Can you work these out from the model? Positions are in its coordinate system, mm. A direction names the side the tool comes from. Round coordinates to 2 decimals unless told otherwise and drop trailing zeros. Loops run counter-clockwise (first coordinate to the right, second up) from the corner with the lowest first, then second, coordinate; pieces in that order, holes last. Notation, with made-up numbers: (-32.75, -5.75) -> (-6.75, -5.75) arc R21 ccw to (-6.75, 27.25) -> close; hole circle Ø10 at (-15.5, 41.25). An arc over 180 degrees is marked (long way). Write item = value, one per line.
from build123d import *

# Parameters (mm, degrees)
GENERAL_SHAPE_DEPTH      = 800
SKETCH5_W                = 1800
SKETCH5_H                = 700
CUT_EXTRUDE2_DEPTH       = 75
SKETCH6_W                = 1300
SKETCH6_H                = 156.02
WEIGHT_REDUCTION_DEPTH   = 1223.94273789
BOSS_EXTRUDE3_DEPTH      = 900
BOSS_EXTRUDE3_DEPTH_BACK = 900
SKETCH8_W                = 50
SKETCH8_H                = 75
BOSS_EXTRUDE4_DEPTH      = 120
BOSS_EXTRUDE5_DEPTH      = 120
CUT_EXTRUDE4_DEPTH       = 740
CUT_EXTRUDE4_DEPTH_BACK  = 40
SKETCH7_R                = 7.5
BOSS_EXTRUDE6_DEPTH      = 25
BOSS_EXTRUDE6_DEPTH_BACK = 25
SKETCH12_R               = 9.525
SKETCH13_W               = 31.75
SKETCH13_H               = 68.5
CUT_EXTRUDE5_DEPTH       = 1371.819167563


with BuildPart() as part:
    # Sketch1 → General shape (new body)
    with BuildSketch(Plane.XY):
        Polygon((-900, 213.515667244), (900, 213.515667244), (900, -67.504332756), (500, -67.504332756), (-500, -67.504332756), (-900, -67.504332756), align=None)
    extrude(amount=GENERAL_SHAPE_DEPTH)

    # Sketch5 → Cut-Extrude2 (cut)
    with BuildSketch(Plane(origin=(0, 213.515667244, 0), x_dir=(1, 0, 0), z_dir=(0, 1, 0))):
        with Locations((0, -400)):
            Rectangle(SKETCH5_W, SKETCH5_H)
    extrude(amount=-CUT_EXTRUDE2_DEPTH, mode=Mode.SUBTRACT)

    # Sketch6 → Weight reduction (cut, through all)
    with BuildSketch(Plane(origin=(0, 0, 0), x_dir=(-1, 0, 0), z_dir=(0, 0, -1))):
        with Locations((0, 10.505667244)):
            Rectangle(SKETCH6_W, SKETCH6_H)
    extrude(amount=-WEIGHT_REDUCTION_DEPTH, mode=Mode.SUBTRACT)

    # Sketch8 → Boss-Extrude3 (add, two sides: drawn at the far end of the back side and taken through both)
    with BuildSketch(Plane(origin=(0, 0, 0), x_dir=(0, 0, -1), z_dir=(1, 0, 0)).offset(-BOSS_EXTRUDE3_DEPTH_BACK)):
        with Locations((-715, 176.015667244)):
            Rectangle(SKETCH8_W, SKETCH8_H)
        with Locations((-85, 176.015667244)):
            Rectangle(SKETCH8_W, SKETCH8_H)
    extrude(amount=BOSS_EXTRUDE3_DEPTH + BOSS_EXTRUDE3_DEPTH_BACK)

    # Sketch9 → Boss-Extrude4 (add)
    with BuildSketch(Plane(origin=(900, 0, 0), x_dir=(0, 0, -1), z_dir=(1, 0, 0))):
        Polygon((-800, 213.515667244), (-750, 213.515667244), (-750, 138.515667244), (-740, 138.515667244), (-740, 213.515667244), (-690, 213.515667244), (-690, 107.495667244), (-110, 107.495667244), (-110, 182.495667244), (-60, 182.495667244), (-60, 107.495667244), (-50, 107.495667244), (-50, 182.495667244), (0, 182.495667244), (0, -67.504332756), (-800, -67.504332756), align=None)
    extrude(amount=BOSS_EXTRUDE4_DEPTH)

    # Sketch10 → Boss-Extrude5 (add)
    with BuildSketch(Plane.ZY.offset(900)):
        Polygon((800, 213.515667244), (750, 213.515667244), (750, 138.515667244), (740, 138.515667244), (740, 213.515667244), (690, 213.515667244), (690, 107.495667244), (110, 107.495667244), (110, 182.495667244), (60, 182.495667244), (60, 107.495667244), (50, 107.495667244), (50, 182.495667244), (0, 182.495667244), (0, -67.504332756), (800, -67.504332756), align=None)
    extrude(amount=BOSS_EXTRUDE5_DEPTH)

    # Sketch7 → Cut-Extrude4 (cut, two sides: drawn at the far end of the back side and taken through both)
    with BuildSketch(Plane(origin=(0, 0, 750), x_dir=(-1, 0, 0), z_dir=(0, 0, -1)).offset(-CUT_EXTRUDE4_DEPTH_BACK)):
        with Locations(Location((-35, 176.015667244, 0), (0, 0, 180))):
            Circle(SKETCH7_R)
        with Locations(Location((-350, 176.015667244, 0), (0, 0, 180))):
            Circle(SKETCH7_R)
        with Locations(Location((-310, 176.015667244, 0), (0, 0, 180))):
            Circle(SKETCH7_R)
        with Locations(Location((10, 176.015667244, 0), (0, 0, 180))):
            Circle(SKETCH7_R)
        with BuildLine():
            Line((960, 168.515667244), (510, 168.515667244))
            ThreePointArc((510, 168.515667244), (502.5, 176.015667244), (510, 183.515667244))
            Line((510, 183.515667244), (960, 183.515667244))
            ThreePointArc((960, 183.515667244), (967.5, 176.015667244), (960, 168.515667244))
        make_face()
        with BuildLine():
            Line((-1000, 183.515667244), (-675, 183.515667244))
            ThreePointArc((-675, 183.515667244), (-667.5, 176.015667244), (-675, 168.515667244))
            Line((-675, 168.515667244), (-1000, 168.515667244))
            ThreePointArc((-1000, 168.515667244), (-1007.5, 176.015667244), (-1000, 183.515667244))
        make_face()
    extrude(amount=CUT_EXTRUDE4_DEPTH + CUT_EXTRUDE4_DEPTH_BACK, mode=Mode.SUBTRACT)

    # Sketch12 → Boss-Extrude6 (add, two sides: drawn at the far end of the back side and taken through both)
    # profile 1 of 2: a face of its own
    with BuildSketch(Plane(origin=(0, 0, 400), x_dir=(-1, 0, 0), z_dir=(0, 0, -1)).offset(-BOSS_EXTRUDE6_DEPTH_BACK)):
        with BuildLine():
            Line((72.5, 138.515667244), (72.5, 194.615667244))
            ThreePointArc((72.5, 194.615667244), (68.868124087, 203.383791331), (60.1, 207.015667244))
            Line((60.1, 207.015667244), (59.9, 207.015667244))
            ThreePointArc((59.9, 207.015667244), (51.131875913, 203.383791331), (47.5, 194.615667244))
            Line((47.5, 194.615667244), (47.5, 138.515667244))
            Line((47.5, 138.515667244), (72.5, 138.515667244))
        make_face()
        with Locations((60, 192.015667244)):
            Circle(SKETCH12_R, mode=Mode.SUBTRACT)
    # profile 2 of 2: a face of its own
    with BuildSketch(Plane(origin=(0, 0, 400), x_dir=(-1, 0, 0), z_dir=(0, 0, -1)).offset(-BOSS_EXTRUDE6_DEPTH_BACK)):
        with BuildLine():
            Line((-345, 138.515667244), (-345, 194.615667244))
            ThreePointArc((-345, 194.615667244), (-348.631875913, 203.383791331), (-357.4, 207.015667244))
            Line((-357.4, 207.015667244), (-357.6, 207.015667244))
            ThreePointArc((-357.6, 207.015667244), (-366.368124087, 203.383791331), (-370, 194.615667244))
            Line((-370, 194.615667244), (-370, 138.515667244))
            Line((-370, 138.515667244), (-345, 138.515667244))
        make_face()
        with Locations((-357.5, 192.015667244)):
            Circle(SKETCH12_R, mode=Mode.SUBTRACT)
    extrude(amount=BOSS_EXTRUDE6_DEPTH + BOSS_EXTRUDE6_DEPTH_BACK)

    # Sketch13 → Cut-Extrude5 (cut, through all)
    with BuildSketch(Plane.ZY.offset(72.5)):
        with Locations((400, 172.765667244)):
            Rectangle(SKETCH13_W, SKETCH13_H)
    extrude(amount=-CUT_EXTRUDE5_DEPTH, mode=Mode.SUBTRACT)


solid = part.part
1. Suppose I cut it at A-A, the plane y = -17.5. List the corners of the cut face in (x, z) for me, and give its area (3 significant figures).
Entries:
outline = (-1020, 0) -> (-650, 0) -> (-650, 800) -> (-1020, 800) -> close; (650, 0) -> (1020, 0) -> (1020, 800) -> (650, 800) -> close
area = 592,000 mm²
2. I need wall thicknesses on line 1 (Z direction, x = 176, y = 144.5); line 2 (X direction, y = 32, z = 575); line 3 (Z direction, x = 715, y = 172). Which ranges of each line are inside material? Lowest first, please. Write a range as [from, to].
Entries:
line_1 = [0, 50], [60, 110], [690, 740], [750, 800]
line_2 = [-1020, -650], [650, 1020]
line_3 = [0, 10], [790, 800]
3. Suppose I cut it at D-D, the plane x = -314.5. List the corners of the cut face in (y, z) for me, and give its area (3 significant figures).
Entries:
outline = (88.52, 0) -> (213.52, 0) -> (213.52, 50) -> (138.52, 50) -> (138.52, 60) -> (213.52, 60) -> (213.52, 110) -> (138.52, 110) -> (138.52, 690) -> (213.52, 690) -> (213.52, 740) -> (138.52, 740) -> (138.52, 750) -> (213.52, 750) -> (213.52, 800) -> (88.52, 800) -> close
area = 55,000 mm²
4. I'm going to push flat-ended pins straight in: pin 1 (4.5 mm diameter, centred on y = 159, z = 378, fed in from +X); pin 2 (9.5 mm diameter, centred on y = 204.5, z = 16.5, fed in from +X); pin 3 (1 mm diameter, centred on x = -743.5, y = 127, fed in from -Z); pin 4 (5 mm diameter, centred on x = -534, z = 682, fed in from -Y). Where does each tip first touch, or does it pass through?
Entries:
pin_1 = 370
pin_2 = 900
pin_3 = 0
pin_4 = 88.52
5. For faces 1 (the flat face through (650, 9, 394)), 2 (the flat face through (840, 183.516, 770)), 3 (the flat face through (14, 175, 740)), which set-ups out of +Z, -Z, +X, -X, +Y, -Y let a thin tool reach every point of the face, with its end or its side?
Entries:
face_1 = +Z, -Z, -Y
face_2 = none
face_3 = +X, -X, +Y
6. Suppose I cut it at C-C, the plane z = 300.5. List the corners of the cut face in (x, y) for me, and give its area (3 significant figures).
Entries:
outline = (-1020, -67.5) -> (-650, -67.5) -> (-650, 88.52) -> (650, 88.52) -> (650, -67.5) -> (1020, -67.5) -> (1020, 107.5) -> (900, 107.5) -> (900, 138.52) -> (-900, 138.52) -> (-900, 107.5) -> (-1020, 107.5) -> close
area = 210,000 mm²
7. Suppose I cut it at B-B, the plane x = 741.5. Count the separate pieces of the cut face and the enclosed holes in it, and give its area (3 significant figures).
Entries:
separate_pieces = 3
enclosed_holes = 0
area = 177,000 mm²
8. We'd pull the mould along Z, two halves only. Please class faces 4 (the flat face through (14, 106, 0)), 5 (the flat face through (-702, 183.516, 85)), 6 (the flat face through (-986, 182.496, 20)): released by +Z, released by -Z, zero draft, split by the parting line, or undercut.
Entries:
face_4 = released by -Z
face_5 = undercut
face_6 = zero draft
